Geometry check sheet. Reference: the model listing, model coordinates, mm. Face numbers are marked on the shaded views. Give positions to 0.01 mm unless a question says otherwise; leave off trailing zeros. Write each loop counter-clockwise with the first axis right and the second up, starting at its lowest first coordinate (ties: lowest second). Pieces come first, ordered by that corner, then holes. Notation, with made-up numbers: (87.5, 48.25) - (117.5, 48.25) arc R23 cw to (117.5, 66.25) - close; hole circle Ø6 at (-21, 47.5). An arc over 180 degrees is marked (long way). Use a Markdown table: item, result.
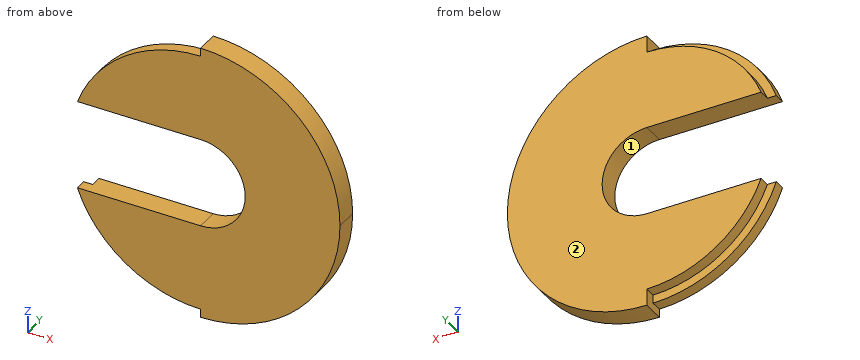
```python
from build123d import *

# Parameters (mm, degrees)
BOSS_EXTRUDE1_DEPTH = 2
BOSS_EXTRUDE2_START = 1
SKETCH1_5_R         = 11.75
BOSS_EXTRUDE2_DEPTH = 1
CUT_EXTRUDE4_DEPTH  = 11
BOSS_EXTRUDE3_DEPTH = 1
BOSS_EXTRUDE4_DEPTH = 1
CUT_EXTRUDE5_START  = 2
CUT_EXTRUDE5_DEPTH  = 1
BOSS_EXTRUDE5_DEPTH = 2


with BuildPart() as part:
    # Sketch1 → Boss-Extrude1 (new body)
    with BuildSketch(Plane(origin=(0, 0, 0), x_dir=(1, 0, 0), z_dir=(0, 1, 0))):
        with BuildLine():
            Line((0, 12.5), (0, 11.75))
            ThreePointArc((0, 11.75), (8.308504679, 8.308504679), (11.75, 0))
            ThreePointArc((11.75, 0), (8.308504679, -8.308504679), (0, -11.75))
            Line((0, -11.75), (0, -12.5))
            ThreePointArc((0, -12.5), (8.838834765, -8.838834765), (12.5, 0))
            ThreePointArc((12.5, 0), (8.838834765, 8.838834765), (0, 12.5))
        make_face()
        with BuildLine():
            Line((0, 11.75), (0, 11.0045))
            ThreePointArc((0, 11.0045), (7.781356574, 7.781356574), (11.0045, 0))
            ThreePointArc((11.0045, 0), (7.781356574, -7.781356574), (0, -11.0045))
            Line((0, -11.0045), (0, -11.75))
            ThreePointArc((0, -11.75), (8.308504679, -8.308504679), (11.75, 0))
            ThreePointArc((11.75, 0), (8.308504679, 8.308504679), (0, 11.75))
        make_face()
    extrude(amount=BOSS_EXTRUDE1_DEPTH)

    # Sketch1<5> → Boss-Extrude2 (add)
    with BuildSketch(Plane(origin=(0, 0, 0), x_dir=(1, 0, 0), z_dir=(0, 1, 0)).offset(BOSS_EXTRUDE2_START)):
        Circle(SKETCH1_5_R)
    extrude(amount=BOSS_EXTRUDE2_DEPTH)

    # Sketch1<8> → Cut-Extrude4 (cut)
    with BuildSketch(Plane(origin=(0, 0, 0), x_dir=(1, 0, 0), z_dir=(0, 1, 0))):
        with BuildLine():
            ThreePointArc((4.0025, 0), (2.830194892, 2.830194892), (0, 4.0025))
            Line((0, 4.0025), (0, -4.0025))
            ThreePointArc((0, -4.0025), (2.830194892, -2.830194892), (4.0025, 0))
        make_face()
        with BuildLine():
            Line((0, -4.0025), (0, 4.0025))
            ThreePointArc((0, 4.0025), (-4.0025, 0), (0, -4.0025))
        make_face()
        with BuildLine():
            ThreePointArc((0, -4.0025), (-4.0025, 0), (0, 4.0025))
            Line((0, 4.0025), (-10.250805529, 4.0025))
            ThreePointArc((-10.250805529, 4.0025), (-11.0045, 0), (-10.250805529, -4.0025))
            Line((-10.250805529, -4.0025), (0, -4.0025))
        make_face()
        with BuildLine():
            ThreePointArc((-10.250805529, -4.0025), (-11.0045, 0), (-10.250805529, 4.0025))
            Line((-10.250805529, 4.0025), (-11.047284451, 4.0025))
            ThreePointArc((-11.047284451, 4.0025), (-11.75, 0), (-11.047284451, -4.0025))
            Line((-11.047284451, -4.0025), (-10.250805529, -4.0025))
        make_face()
    extrude(amount=CUT_EXTRUDE4_DEPTH, mode=Mode.SUBTRACT)

    # Sketch1<9> → Boss-Extrude3 (add)
    with BuildSketch(Plane(origin=(0, 0, 0), x_dir=(1, 0, 0), z_dir=(0, 1, 0))):
        with BuildLine():
            Line((0, 11.0045), (0, 4.0025))
            ThreePointArc((0, 4.0025), (2.830194892, 2.830194892), (4.0025, 0))
            ThreePointArc((4.0025, 0), (2.830194892, -2.830194892), (0, -4.0025))
            Line((0, -4.0025), (0, -11.0045))
            ThreePointArc((0, -11.0045), (7.781356574, -7.781356574), (11.0045, 0))
            ThreePointArc((11.0045, 0), (7.781356574, 7.781356574), (0, 11.0045))
        make_face()
    extrude(amount=BOSS_EXTRUDE3_DEPTH)

    # Sketch1<10> → Boss-Extrude4 (add)
    with BuildSketch(Plane(origin=(0, 0, 0), x_dir=(1, 0, 0), z_dir=(0, 1, 0))):
        with BuildLine():
            Line((-10.250805529, 4.0025), (0, 4.0025))
            Line((0, 4.0025), (0, 11.0045))
            ThreePointArc((0, 11.0045), (-6.206992388, 9.08692829), (-10.250805529, 4.0025))
        make_face()
        with BuildLine():
            Line((0, -11.0045), (0, -4.0025))
            Line((0, -4.0025), (-10.250805529, -4.0025))
            ThreePointArc((-10.250805529, -4.0025), (-6.206992388, -9.08692829), (0, -11.0045))
        make_face()
        with BuildLine():
            Line((0, -11.75), (0, -11.0045))
            ThreePointArc((0, -11.0045), (-6.206992388, -9.08692829), (-10.250805529, -4.0025))
            Line((-10.250805529, -4.0025), (-11.047284451, -4.0025))
            ThreePointArc((-11.047284451, -4.0025), (-6.746596364, -9.620079911), (0, -11.75))
        make_face()
        with BuildLine():
            ThreePointArc((-10.250805529, 4.0025), (-6.206992388, 9.08692829), (0, 11.0045))
            Line((0, 11.0045), (0, 11.75))
            ThreePointArc((0, 11.75), (-6.746596364, 9.620079911), (-11.047284451, 4.0025))
            Line((-11.047284451, 4.0025), (-10.250805529, 4.0025))
        make_face()
    extrude(amount=BOSS_EXTRUDE4_DEPTH)

    # Sketch1<11> → Cut-Extrude5 (cut)
    with BuildSketch(Plane(origin=(0, 0, 0), x_dir=(1, 0, 0), z_dir=(0, 1, 0)).offset(CUT_EXTRUDE5_START)):
        with BuildLine():
            Line((-10.250805529, 4.0025), (0, 4.0025))
            Line((0, 4.0025), (0, 11.0045))
            ThreePointArc((0, 11.0045), (-6.206992388, 9.08692829), (-10.250805529, 4.0025))
        make_face()
        with BuildLine():
            ThreePointArc((-10.250805529, 4.0025), (-6.206992388, 9.08692829), (0, 11.0045))
            Line((0, 11.0045), (0, 11.75))
            ThreePointArc((0, 11.75), (-6.746596364, 9.620079911), (-11.047284451, 4.0025))
            Line((-11.047284451, 4.0025), (-10.250805529, 4.0025))
        make_face()
        with BuildLine():
            Line((0, -11.0045), (0, -4.0025))
            Line((0, -4.0025), (-10.250805529, -4.0025))
            ThreePointArc((-10.250805529, -4.0025), (-6.206992388, -9.08692829), (0, -11.0045))
        make_face()
        with BuildLine():
            Line((0, -11.75), (0, -11.0045))
            ThreePointArc((0, -11.0045), (-6.206992388, -9.08692829), (-10.250805529, -4.0025))
            Line((-10.250805529, -4.0025), (-11.047284451, -4.0025))
            ThreePointArc((-11.047284451, -4.0025), (-6.746596364, -9.620079911), (0, -11.75))
        make_face()
    extrude(amount=-CUT_EXTRUDE5_DEPTH, mode=Mode.SUBTRACT)

    # Sketch1<12> → Boss-Extrude5 (add)
    with BuildSketch(Plane(origin=(0, 0, 0), x_dir=(1, 0, 0), z_dir=(0, 1, 0))):
        with BuildLine():
            Line((0, -11.0045), (0, -4.0025))
            Line((0, -4.0025), (-10.250805529, -4.0025))
            ThreePointArc((-10.250805529, -4.0025), (-6.206992388, -9.08692829), (0, -11.0045))
        make_face()
        with BuildLine():
            Line((-10.250805529, 4.0025), (0, 4.0025))
            Line((0, 4.0025), (0, 11.0045))
            ThreePointArc((0, 11.0045), (-6.206992388, 9.08692829), (-10.250805529, 4.0025))
        make_face()
    extrude(amount=BOSS_EXTRUDE5_DEPTH)


solid = part.part
```
1) Depth check by flat-ended pin: P1, Ø1, axis at x = -3, y = 0.5, coming from the +Z side; P2, Ø1, axis at x = -6.5, y = 1, coming from the -Z side; P3, Ø3, axis at x = 1, z = -1.5, coming from the -Y side. Enter the tip coordinate at first touch or a pass-through.
Working result:
| item | result |
|---|---|
| P1 | stops at z = 11.48 |
| P2 | stops at z = -10.1 |
| P3 | passes through |
2) Material ranges on L1, parallel to Z at x = -0.25, y = 1.45; L2, parallel to Z at x = -3.5, y = 1.8; L3, parallel to X at y = 0.7, z = -5.5, recorded low to high. Write a range as from..to.
Working result:
| item | result |
|---|---|
| L1 | z = -11..-4, 4..11 |
| L2 | z = -10.43..-4, 4..10.43 |
| L3 | x = -10.38..11.22 |
3) Section check D-D on x = -1.5. Record the boundary of the cut face in (y, z), then the cut area to 3 significant figures.
Working result:
| item | result |
|---|---|
| outline | (0, -11.65) - (1, -11.65) - (1, -10.9) - (2, -10.9) - (2, -4) - (0, -4) - close; (0, 4) - (2, 4) - (2, 10.9) - (1, 10.9) - (1, 11.65) - (0, 11.65) - close |
| area | 29.1 mm² |
4) Section check C-C on z = -6. Record the boundary of the cut face in (x, y), then the cut area to 3 significant figures.
Working result:
| item | result |
|---|---|
| outline | (-10.1, 0) - (10.97, 0) - (10.97, 2) - (-9.22, 2) - (-9.22, 1) - (-10.1, 1) - close |
| area | 41.3 mm² |
5) Section check A-A on x = 2. Record the boundary of the cut face in (y, z), then the cut area to 3 significant figures.
Working result:
| item | result |
|---|---|
| outline | (0, -12.34) - (2, -12.34) - (2, -3.47) - (0, -3.47) - close; (0, 3.47) - (2, 3.47) - (2, 12.34) - (0, 12.34) - close |
| area | 35.5 mm² |
6) Mould release check, pull along Z, two halves, no side actions. Record for the marked faces 1 and 2: pulls with the +Z half, pulls with the -Z half, needs draft (parallel to the pull), parting line crosses it, or undercut.
Working result:
| item | result |
|---|---|
| face 1 | undercut |
| face 2 | needs draft |
